from build123d import *

# Parameters (mm, degrees)
SKETCH_W           = 40
SKETCH_H           = 40
PAD_DEPTH          = 17
SKETCH001_R        = 7
PAD001_DEPTH       = 8
SKETCH002_R        = 4
POCKET_DEPTH       = 25
CYLINDER_R         = 6
CYLINDER_DEPTH     = 1
PAD002_DEPTH       = 8.4
SKETCH004_R        = 4.2
POCKET001_DEPTH    = 7
PAD003_DEPTH       = 8.4
SKETCH006_R        = 4.2
POCKET002_DEPTH    = 7
POCKET003_DEPTH    = 8
POLARPATTERN_COUNT = 4
FILLET_R           = 1
FILLET001_R        = 1.5
FILLET002_R        = 0.6


with BuildPart() as part:
    # Sketch → Pad (new body)
    with BuildSketch(Plane.XY):
        Rectangle(SKETCH_W, SKETCH_H)
    extrude(amount=PAD_DEPTH)

    # Sketch001 (on Face6 of Pad) → Pad001 (join)
    with BuildSketch(Plane.XY.offset(17)):
        Circle(SKETCH001_R)
    extrude(amount=PAD001_DEPTH)

    # Sketch002 (on Face8 of Pad001) → Pocket (cut)
    with BuildSketch(Plane.XY.offset(25)):
        Circle(SKETCH002_R)
    extrude(amount=-POCKET_DEPTH, mode=Mode.SUBTRACT)

    # Cylinder → Cylinder (cut)
    with BuildSketch(Plane.XY.offset(24)):
        Circle(CYLINDER_R)
    extrude(amount=CYLINDER_DEPTH, mode=Mode.SUBTRACT)

    # Sketch003 → Pad002 (join, symmetric)
    with BuildSketch(Plane.XZ):
        Polygon((20, 17), (27, 0), (27, -15), (20, -15), align=None)
    extrude(amount=PAD002_DEPTH, both=True)

    # Sketch004 (on Face16 of Pad002) → Pocket001 (cut)
    with BuildSketch(Plane(origin=(27, 0, 24), x_dir=(0, 1, 0), z_dir=(1, 0, 0))):
        with Locations((0, -32)):
            Circle(SKETCH004_R)
    extrude(amount=-POCKET001_DEPTH, mode=Mode.SUBTRACT)

    # Sketch005 → Pad003 (join, symmetric)
    with BuildSketch(Plane.YZ):
        Polygon((-20, 17), (-27, 0), (-27, -15), (-20, -15), align=None)
    extrude(amount=PAD003_DEPTH, both=True)

    # Sketch006 (on Face17 of Pad003) → Pocket002 (cut)
    with BuildSketch(Plane(origin=(0, -27, 24), x_dir=(1, 0, 0), z_dir=(0, -1, 0))):
        with Locations((0, -32)):
            Circle(SKETCH006_R)
    extrude(amount=-POCKET002_DEPTH, mode=Mode.SUBTRACT)

    # Sketch007 (on Face4 of Pocket002) → Pocket003 (cut)
    with BuildSketch(Plane(origin=(0, 0, 0), x_dir=(1, 0, 0), z_dir=(0, 0, -1))):
        with BuildLine():
            ThreePointArc((5.656854, 2), (4.242641, 4.242641), (2, 5.656854))
            Line((2, 18), (2, 5.656854))
            Line((2, 18), (18, 18))
            Line((18, 18), (18, 2))
            Line((18, 2), (5.656854, 2))
        make_face()
    pocket003 = extrude(amount=-POCKET003_DEPTH, mode=Mode.SUBTRACT)

    # PolarPattern: Pocket003 ×4 about axis
    polarpattern_axis = Axis((0, 0, 0), (0, 0, -1))
    for i in range(1, POLARPATTERN_COUNT):
        add(pocket003.rotate(polarpattern_axis, i * 360 / POLARPATTERN_COUNT), mode=Mode.SUBTRACT)

    # Fillet
    fillet_edges = [part.edges().sort_by_distance(p)[0] for p in [
        (5.656854, -2, 4),
        (2, -5.656854, 4),
        (2, -18, 4),
        (18, -18, 4),
        (18, -2, 4),
        (5.656854, 2, 4),
        (18, 2, 4),
        (18, 18, 4),
        (2, 18, 4),
        (2, 5.656854, 4),
        (-2, 5.656854, 4),
        (-18, 2, 4),
        (-18, 18, 4),
        (-2, 18, 4),
        (-5.656854, 2, 4),
        (-5.656854, -2, 4),
        (-2, -5.656854, 4),
        (-2, -18, 4),
        (-18, -18, 4),
        (-18, -2, 4),
    ]]
    fillet(fillet_edges, radius=FILLET_R)

    # Fillet001
    fillet001_edges = [part.edges().sort_by_distance(p)[0] for p in [
        (20, 20, 8.5),
        (-20, 20, 8.5),
        (-20, -20, 8.5),
        (20, -20, 8.5),
    ]]
    fillet(fillet001_edges, radius=FILLET001_R)

    # Fillet002
    fillet002_edges = [part.edges().sort_by_distance(p)[0] for p in [
        (23.5, -8.4, -15),
        (23.5, 8.4, -15),
        (8.4, -23.5, -15),
        (-8.4, -23.5, -15),
        (0, -27, -15),
        (0, -20, -15),
        (27, 0, -15),
        (20, 0, -15),
        (27, -8.4, -7.5),
        (20, -8.4, -7.5),
        (27, 8.4, -7.5),
        (20, 8.4, -7.5),
        (8.4, -20, -7.5),
        (8.4, -27, -7.5),
        (-8.4, -20, -7.5),
        (-8.4, -27, -7.5),
    ]]
    fillet(fillet002_edges, radius=FILLET002_R)


solid = part.part
The listing builds one solid part. Answer for the finished solid, in the listing's coordinates (mm). A direction names the side the tool comes from. Coordinates: 2 decimals unless noted, no trailing zeros. Loops run counter-clockwise (first coordinate to the right, second up) from the corner with the lowest first, then second, coordinate; pieces in that order, holes last. Notation, with made-up numbers: (-12, 42) -> (18, 42) arc R27 cw to (18, 76) -> close; hole circle Ø5 at (-19.5, -32). An arc over 180 degrees is marked (long way). Answer in a Markdown table with one row per item. Add a question column.
1. The part is cut by section D-D, the plane x = -16. Write down the section's boundary in (y, z), then the cut area to 3 significant figures.
2. The part is cut by section A-A, the plane z = -8. Write down the section's boundary in (x, y), then the cut area to 3 significant figures.
3. The part is cut by section B-B, the plane y = 0. Write down the section's boundary in (x, z), then the cut area to 3 significant figures.
4. The part is cut by section C-C, the plane x = 0. Write down the section's boundary in (y, z).
5. Consider line 1 (X direction, y = -11.5, z = 3); line 2 (Y direction, x = 0, z = 24.45). Determine where each line is inside the solid, lowest interval first. Write a range as [from, to].
6. Determine the mould class of faces 1 (the flat face through (-1.42, -3.92, 24)), 2 (the cylindrical face through (-0.867, -3.905, 12.168)), 3 (the cylindrical face through (-0.91, -23.55, -12.1)) for opening direction Z: +Z half, -Z half, draft (parallel to the pull), parting line (faces both ways), or undercut.
7. For faces 4 (the flat face through (8.4, -23, -2)), 5 (the cylindrical face through (-19.57, 19.55, 8.62)), 6 (the flat face through (2, -20, -4)), 7 (the flat face through (18, 10, 4)), 8 (the flat face through (20, 13, 8)), determine the directions among +Z, -Z, +X, -X, +Y, -Y from which every point of the face is accessible in a straight line to the end or side of a thin tool.
8. Flat-ended cylindrical pins translate along their axes: P1, Ø3, axis at y = -17.5, z = 10.5, coming from the +X side; P2, Ø6, axis at x = 15.5, y = -13, coming from the -Z side; P3, Ø4.5, axis at x = 0, z = -4.5, coming from the +Y side; P4, Ø5, axis at x = 20, z = -1, coming from the +Y side. Find the tip coordinate at first contact, or state that the pin passes through.
Answer below:
| question | item | result |
|---|---|---|
| 1 | outline | (-20, 0) -> (-18, 0) -> (-18, 8) -> (-2, 8) -> (-2, 0) -> (2, 0) -> (2, 8) -> (18, 8) -> (18, 0) -> (20, 0) -> (20, 17) -> (-20, 17) -> close |
| 1 | area | 424 mm2 |
| 2 | outline | (-8.4, -26.4) arc R0.6 ccw to (-7.8, -27) -> (-4.2, -27) -> (-4.2, -20) -> (-7.8, -20) arc R0.6 ccw to (-8.4, -20.6) -> close; (4.2, -27) -> (7.8, -27) arc R0.6 ccw to (8.4, -26.4) -> (8.4, -20.6) arc R0.6 ccw to (7.8, -20) -> (4.2, -20) -> close; (20, -7.8) arc R0.6 ccw to (20.6, -8.4) -> (26.4, -8.4) arc R0.6 ccw to (27, -7.8) -> (27, -4.2) -> (20, -4.2) -> close; (20, 4.2) -> (27, 4.2) -> (27, 7.8) arc R0.6 ccw to (26.4, 8.4) -> (20.6, 8.4) arc R0.6 ccw to (20, 7.8) -> close |
| 2 | area | 117 mm2 |
| 3 | outline | (-20, 0) -> (-4, 0) -> (-4, 24) -> (-6, 24) -> (-6, 25) -> (-7, 25) -> (-7, 17) -> (-20, 17) -> close; (4, 0) -> (20, 0) -> (20, -3.8) -> (27, -3.8) -> (27, 0) -> (20, 17) -> (7, 17) -> (7, 25) -> (6, 25) -> (6, 24) -> (4, 24) -> close; (20, -14.4) arc R0.6 ccw to (20.6, -15) -> (26.4, -15) arc R0.6 ccw to (27, -14.4) -> (27, -12.2) -> (20, -12.2) -> close |
| 3 | area | 694 mm2 |
| 4 | outline | (-27, -14.4) arc R0.6 ccw to (-26.4, -15) -> (-20.6, -15) arc R0.6 ccw to (-20, -14.4) -> (-20, -12.2) -> (-27, -12.2) -> close; (-27, -3.8) -> (-20, -3.8) -> (-20, 0) -> (-4, 0) -> (-4, 24) -> (-6, 24) -> (-6, 25) -> (-7, 25) -> (-7, 17) -> (-20, 17) -> (-27, 0) -> close; (4, 0) -> (20, 0) -> (20, 17) -> (7, 17) -> (7, 25) -> (6, 25) -> (6, 24) -> (4, 24) -> close |
| 5 | line 1 | [-20, -18], [-2, 2], [18, 20] |
| 5 | line 2 | [-7, -6], [6, 7] |
| 6 | face 1 | +Z half |
| 6 | face 2 | draft |
| 6 | face 3 | undercut |
| 7 | face 4 | +Z, -Z, +X, -Y |
| 7 | face 5 | +Z, -Z, -X, +Y |
| 7 | face 6 | -Z, +X, -X, +Y |
| 7 | face 7 | -Z |
| 7 | face 8 | +Z, -Z, +X, +Y |
| 8 | P1 | x = 20 |
| 8 | P2 | z = 0 |
| 8 | P3 | y = -20 |
| 8 | P4 | y = 20 |
